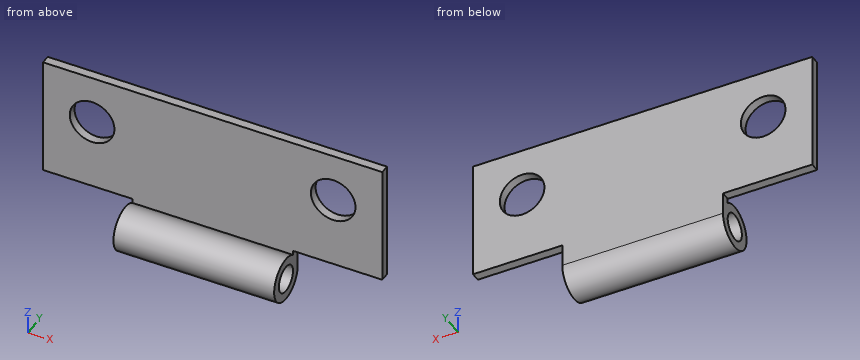
from build123d import *

# Parameters (mm, degrees)
SKETCH3_R           = 1.5
BOSS_EXTRUDE2_DEPTH = 38
SKETCH4_W           = 10
SKETCH4_H           = 5
CUT_EXTRUDE1_DEPTH  = 6
SKETCH5_R           = 2.5
CUT_EXTRUDE2_DEPTH  = 6


with BuildPart() as part:
    # Sketch3 → Boss-Extrude2 (new body)
    with BuildSketch(Plane(origin=(0, 0, 0), x_dir=(0, 0, -1), z_dir=(1, 0, 0))):
        with BuildLine():
            Line((16, 1), (0, 1))
            Line((0, 1), (0, 0))
            Line((0, 0), (14, 0))
            ThreePointArc((14, 0), (17.118033989, -3.736067977), (16, 1))
        make_face()
        with Locations((16, -1.5)):
            Circle(SKETCH3_R, mode=Mode.SUBTRACT)
    extrude(amount=BOSS_EXTRUDE2_DEPTH)

    # Sketch4 → Cut-Extrude1 (cut, through all)
    with BuildSketch(Plane(origin=(0, 1, 0), x_dir=(1, 0, 0), z_dir=(0, 1, 0))):
        with Locations((33, 16)):
            Rectangle(SKETCH4_W, SKETCH4_H)
        with Locations((5, 16)):
            Rectangle(SKETCH4_W, SKETCH4_H)
    extrude(amount=-CUT_EXTRUDE1_DEPTH, mode=Mode.SUBTRACT)

    # Sketch5 → Cut-Extrude2 (cut, through all)
    with BuildSketch(Plane(origin=(0, 1, 0), x_dir=(1, 0, 0), z_dir=(0, 1, 0))):
        with Locations((5.5, 5.5)):
            Circle(SKETCH5_R)
        with Locations((32.5, 5.5)):
            Circle(SKETCH5_R)
    extrude(amount=-CUT_EXTRUDE2_DEPTH, mode=Mode.SUBTRACT)


solid = part.part
Geometry check sheet. Reference: the model listing, model coordinates, mm. Round coordinates to 2 decimals unless told otherwise and drop trailing zeros. Order: outer loops, then holes, each group sorted by start corner. A loop starts at its lowest first (then second) coordinate and runs counter-clockwise, first axis right, second up. Notation, with made-up numbers: M -35.5,-10 L -13.5,-10 A21 ccw -13.5,27 Z; hole C 64.5,86.25 d3. An arc over 180 degrees is marked long. Answer in a Markdown table with one row per item. Add a question column.
Item 1: Material ranges on L1, parallel to X at y = 0.45, z = -5.5; L2, parallel to Y at x = 23, z = -16; L3, parallel to Z at x = 32.5, y = 0.4, recorded low to high. Write a range as [from, to].
Item 2: Depth check by flat-ended pin: pin 1 Ø2.5 at (y, z) = (-2, -15) entering from +X; pin 2 Ø3 at (x, z) = (24.5, -11.5) entering from -Y; pin 3 Ø0.5 at (x, y) = (7, 0.5) entering from -Z; pin 4 Ø4 at (x, z) = (32.5, -5.5) entering from +Y. Enter the tip coordinate at first touch or a pass-through.
Item 3: Sectioned sample at D-D, the plane x = 24.5. Enter the section's corners in (y, z).
Item 4: Sectioned sample at C-C, the plane y = -1.5. Enter the section's corners in (x, z), plus the area to 3 significant figures.
Item 5: Sectioned sample at B-B, the plane x = 32.5. Enter the section's corners in (y, z), plus the area to 3 significant figures.
Item 6: Sectioned sample at A-A, the plane z = -5.5. Enter the section's corners in (x, y), plus the area to 3 significant figures.
Filled in:
| question | item | result |
|---|---|---|
| 1 | L1 | x = [0, 3], [8, 30], [35, 38] |
| 1 | L2 | y = [-4, -3], [0, 1] |
| 1 | L3 | z = [-13.5, -8], [-3, 0] |
| 2 | pin 1 | stops at x = 28 |
| 2 | pin 2 | stops at y = 0 |
| 2 | pin 3 | stops at z = -13.5 |
| 2 | pin 4 | passes through |
| 3 | outline | M 0,-14 A2.5 ccw long 1,-16 L 1,0 L 0,0 Z; hole C -1.5,-16 d3 |
| 4 | outline | M 10,-18.5 L 28,-18.5 L 28,-17.5 L 10,-17.5 Z; M 10,-14.5 L 28,-14.5 L 28,-13.5 L 10,-13.5 Z |
| 4 | area | 36.0 mm² |
| 5 | outline | M 0,-13.5 L 1,-13.5 L 1,-8 L 0,-8 Z; M 0,-3 L 1,-3 L 1,0 L 0,0 Z |
| 5 | area | 8.50 mm² |
| 6 | outline | M 0,0 L 3,0 L 3,1 L 0,1 Z; M 8,0 L 30,0 L 30,1 L 8,1 Z; M 35,0 L 38,0 L 38,1 L 35,1 Z |
| 6 | area | 28.0 mm² |
